Design review of the part built by this model. Coordinates are the model's own, in mm. Face numbers are marked on the shaded views. Round coordinates to 2 decimals unless told otherwise and drop trailing zeros. Order: outer loops, then holes, each group sorted by start corner. A loop starts at its lowest first (then second) coordinate and runs counter-clockwise, first axis right, second up. Notation, with made-up numbers: (26, 31) - (42, 31) arc R20 ccw to (42, 37) - close; hole circle Ø10 at (-32, 58). An arc over 180 degrees is marked (long way). Answer as a JSON object with one key per item and string values. Group by question number.
from build123d import *
from build123d import SkipClean  # not in build123d's __all__

# Parameters (mm, degrees)
F0_R      = 6.35
F1_DEPTH  = 25.4
F2_R      = 6.35
F3_DEPTH  = 25.4
F4_DEPTH  = 5.08
F5_DEPTH  = 8.89
F6_DEPTH  = 20.32
F7_DEPTH  = 10.16
F8_DEPTH  = 5.08
F9_DEPTH  = 13.97
F10_DEPTH = 3.81
F11_W     = 3.81
F11_H     = 6.35
F12_DEPTH = 6.35
F17_DEPTH = 2.032
F18_DEPTH = 2.032


with BuildPart() as f1:
    # F0 (on Front) → F1 (new body)
    with BuildSketch(Plane.XZ):
        with BuildLine():
            ThreePointArc((42.0866659097, -2.2684633732), (38.3669220307, 6.7117927479), (29.3866659097, 10.4315366268))
            ThreePointArc((29.3866659097, 10.4315366268), (20.4064097886, 6.7117927479), (16.6866659097, -2.2684633732))
            ThreePointArc((16.6866659097, -2.2684633732), (20.4064097886, -11.2487194943), (29.3866659097, -14.9684633732))
            ThreePointArc((29.3866659097, -14.9684633732), (38.3669220307, -11.2487194943), (42.0866659097, -2.2684633732))
        make_face()
        with Locations((29.3866659097, -2.2684633732)):
            Circle(F0_R, mode=Mode.SUBTRACT)
        with Locations((29.3866659097, -2.2684633732)):
            Circle(F0_R)
        with BuildLine():
            Line((92.8866659097, 10.4315366268), (29.3866659097, 10.4315366268))
            ThreePointArc((29.3866659097, 10.4315366268), (38.3669220307, 6.7117927479), (42.0866659097, -2.2684633732))
            ThreePointArc((42.0866659097, -2.2684633732), (38.3669220307, -11.2487194943), (29.3866659097, -14.9684633732))
            Line((29.3866659097, -14.9684633732), (92.8866659097, -14.9684633732))
            Line((92.8866659097, -14.9684633732), (92.8866659097, 10.4315366268))
        make_face()
    extrude(amount=-F1_DEPTH)

    # F2 (on face) → F3 (cut, through all)
    with BuildSketch(Plane(origin=(0, 25.4, 0), x_dir=(-1, 0, 0), z_dir=(0, 1, 0))):
        with BuildLine():
            ThreePointArc((-29.3866659097, -14.9684633732), (-42.0866659097, -2.2684633732), (-29.3866659097, 10.4315366268))
            Line((-29.3866659097, 10.4315366268), (-92.8866659097, 10.4315366268))
            Line((-92.8866659097, 10.4315366268), (-92.8866659097, -14.9684633732))
            Line((-92.8866659097, -14.9684633732), (-29.3866659097, -14.9684633732))
        make_face()
        with Locations((-29.3866659097, -2.2684633732)):
            Circle(F2_R)
    with SkipClean():  # cleaning this boolean's faces spoils the solid; the shape is the same uncleaned
        extrude(amount=-F3_DEPTH, mode=Mode.SUBTRACT)

    # F2 (on face) → F4 (join)
    with BuildSketch(Plane(origin=(0, 25.4, 0), x_dir=(-1, 0, 0), z_dir=(0, 1, 0))):
        with BuildLine():
            ThreePointArc((-29.3866659097, -14.9684633732), (-42.0866659097, -2.2684633732), (-29.3866659097, 10.4315366268))
            Line((-29.3866659097, 10.4315366268), (-92.8866659097, 10.4315366268))
            Line((-92.8866659097, 10.4315366268), (-92.8866659097, -14.9684633732))
            Line((-92.8866659097, -14.9684633732), (-29.3866659097, -14.9684633732))
        make_face()
    extrude(amount=-F4_DEPTH)

    # F2 (on face) → F5 (join)
    with BuildSketch(Plane(origin=(0, 25.4, 0), x_dir=(-1, 0, 0), z_dir=(0, 1, 0))):
        with Locations((-29.3866659097, -2.2684633732)):
            Circle(F2_R)
    extrude(amount=-F5_DEPTH)

    # F2 (on face) → F6 (join)
    with BuildSketch(Plane(origin=(0, 25.4, 0), x_dir=(-1, 0, 0), z_dir=(0, 1, 0))):
        with BuildLine():
            ThreePointArc((-29.3866659097, -14.9684633732), (-42.0866659097, -2.2684633732), (-29.3866659097, 10.4315366268))
            Line((-29.3866659097, 10.4315366268), (-92.8866659097, 10.4315366268))
            Line((-92.8866659097, 10.4315366268), (-92.8866659097, -14.9684633732))
            Line((-92.8866659097, -14.9684633732), (-29.3866659097, -14.9684633732))
        make_face()
        with Locations((-29.3866659097, -2.2684633732)):
            Circle(F2_R)
    extrude(amount=-F6_DEPTH)

    # F7 (cut): a face of the model
    f7_faces = [f1.faces().sort_by_distance(p)[0] for p in [
        (29.3866659097, 0, 10.072326382),
    ]]
    extrude(f7_faces, amount=-F7_DEPTH, mode=Mode.SUBTRACT)

    # F8 (cut): a face of the model
    f8_faces = [f1.faces().sort_by_distance(p)[0] for p in [
        (66.0488875518, 5.08, -2.2684633732),
    ]]
    extrude(f8_faces, amount=-F8_DEPTH, mode=Mode.SUBTRACT)

    # F0 (on Front) → F9 (cut)
    with BuildSketch(Plane.XZ):
        with Locations((29.3866659097, -2.2684633732)):
            Circle(F0_R)
    extrude(amount=-F9_DEPTH, mode=Mode.SUBTRACT)

    # F2 (on face) → F10 (cut)
    with BuildSketch(Plane(origin=(0, 25.4, 0), x_dir=(-1, 0, 0), z_dir=(0, 1, 0))):
        with Locations((-29.3866659097, -2.2684633732)):
            Circle(F2_R)
    extrude(amount=-F10_DEPTH, mode=Mode.SUBTRACT)

    # F11 (on face) → F12 (join)
    with BuildSketch(Plane.YZ.offset(92.8866659097)):
        with Locations((12.065, 7.2565366268)):
            Rectangle(F11_W, F11_H)
        with Locations((23.495, 7.2565366268)):
            Rectangle(F11_W, F11_H)
        with Locations((23.495, -11.7934633732)):
            Rectangle(F11_W, F11_H)
        with Locations((12.065, -11.7934633732)):
            Rectangle(F11_W, F11_H)
    extrude(amount=F12_DEPTH)

    # F15 (on face) + F13 (on face) → F17 (join)
    with BuildSketch(Plane(origin=(0, 13.97, 0), x_dir=(-1, 0, 0), z_dir=(0, 1, 0))):
        with BuildLine():
            Line((-96.0616659097, -11.7934633732), (-94.1566659097, -11.7934633732))
            ThreePointArc((-94.1566659097, -11.7934633732), (-94.7146274915, -10.446424955), (-96.0616659097, -9.8884633732))
            Line((-96.0616659097, -9.8884633732), (-96.0616659097, -11.7934633732))
        make_face()
        with BuildLine():
            Line((-97.9666659097, -11.7934633732), (-96.0616659097, -11.7934633732))
            Line((-96.0616659097, -11.7934633732), (-96.0616659097, -9.8884633732))
            ThreePointArc((-96.0616659097, -9.8884633732), (-97.4087043278, -10.446424955), (-97.9666659097, -11.7934633732))
        make_face()
        with BuildLine():
            Line((-96.0616659097, -13.6984633732), (-96.0616659097, -11.7934633732))
            Line((-96.0616659097, -11.7934633732), (-97.9666659097, -11.7934633732))
            ThreePointArc((-97.9666659097, -11.7934633732), (-97.4087043278, -13.1405017913), (-96.0616659097, -13.6984633732))
        make_face()
        with BuildLine():
            ThreePointArc((-96.0616659097, -13.6984633732), (-94.7146274915, -13.1405017913), (-94.1566659097, -11.7934633732))
            Line((-94.1566659097, -11.7934633732), (-96.0616659097, -11.7934633732))
            Line((-96.0616659097, -11.7934633732), (-96.0616659097, -13.6984633732))
        make_face()
    with BuildSketch(Plane(origin=(0, 13.97, 0), x_dir=(-1, 0, 0), z_dir=(0, 1, 0))):
        with BuildLine():
            Line((-96.0616659097, 7.2565366268), (-96.0616659097, 9.1615366268))
            ThreePointArc((-96.0616659097, 9.1615366268), (-97.4087043278, 8.603575045), (-97.9666659097, 7.2565366268))
            Line((-97.9666659097, 7.2565366268), (-96.0616659097, 7.2565366268))
        make_face()
        with BuildLine():
            Line((-96.0616659097, 7.2565366268), (-94.1566659097, 7.2565366268))
            ThreePointArc((-94.1566659097, 7.2565366268), (-94.7146274915, 8.603575045), (-96.0616659097, 9.1615366268))
            Line((-96.0616659097, 9.1615366268), (-96.0616659097, 7.2565366268))
        make_face()
        with BuildLine():
            ThreePointArc((-97.9666659097, 7.2565366268), (-97.4087043278, 5.9094982087), (-96.0616659097, 5.3515366268))
            Line((-96.0616659097, 5.3515366268), (-96.0616659097, 7.2565366268))
            Line((-96.0616659097, 7.2565366268), (-97.9666659097, 7.2565366268))
        make_face()
        with BuildLine():
            ThreePointArc((-96.0616659097, 5.3515366268), (-94.7146274915, 5.9094982087), (-94.1566659097, 7.2565366268))
            Line((-94.1566659097, 7.2565366268), (-96.0616659097, 7.2565366268))
            Line((-96.0616659097, 7.2565366268), (-96.0616659097, 5.3515366268))
        make_face()
    extrude(amount=F17_DEPTH)

    # F14 (on face) + F16 (on face) → F18 (join)
    with BuildSketch(Plane.XZ.offset(-21.59)):
        with BuildLine():
            Line((96.0616659097, 7.2565366268), (96.0616659097, 9.1615366268))
            ThreePointArc((96.0616659097, 9.1615366268), (94.7146274915, 8.603575045), (94.1566659097, 7.2565366268))
            Line((94.1566659097, 7.2565366268), (96.0616659097, 7.2565366268))
        make_face()
        with BuildLine():
            Line((96.0616659097, 7.2565366268), (97.9666659097, 7.2565366268))
            ThreePointArc((97.9666659097, 7.2565366268), (97.4087043278, 8.603575045), (96.0616659097, 9.1615366268))
            Line((96.0616659097, 9.1615366268), (96.0616659097, 7.2565366268))
        make_face()
        with BuildLine():
            ThreePointArc((96.0616659097, 5.3515366268), (97.4087043278, 5.9094982087), (97.9666659097, 7.2565366268))
            Line((97.9666659097, 7.2565366268), (96.0616659097, 7.2565366268))
            Line((96.0616659097, 7.2565366268), (96.0616659097, 5.3515366268))
        make_face()
        with BuildLine():
            ThreePointArc((94.1566659097, 7.2565366268), (94.7146274915, 5.9094982087), (96.0616659097, 5.3515366268))
            Line((96.0616659097, 5.3515366268), (96.0616659097, 7.2565366268))
            Line((96.0616659097, 7.2565366268), (94.1566659097, 7.2565366268))
        make_face()
    with BuildSketch(Plane.XZ.offset(-21.59)):
        with BuildLine():
            Line((94.1566659097, -11.7934633732), (96.0616659097, -11.7934633732))
            Line((96.0616659097, -11.7934633732), (96.0616659097, -9.8884633732))
            ThreePointArc((96.0616659097, -9.8884633732), (94.7146274915, -10.446424955), (94.1566659097, -11.7934633732))
        make_face()
        with BuildLine():
            Line((96.0616659097, -9.8884633732), (96.0616659097, -11.7934633732))
            Line((96.0616659097, -11.7934633732), (97.9666659097, -11.7934633732))
            ThreePointArc((97.9666659097, -11.7934633732), (97.4087043278, -10.446424955), (96.0616659097, -9.8884633732))
        make_face()
        with BuildLine():
            Line((96.0616659097, -11.7934633732), (96.0616659097, -13.6984633732))
            ThreePointArc((96.0616659097, -13.6984633732), (97.4087043278, -13.1405017913), (97.9666659097, -11.7934633732))
            Line((97.9666659097, -11.7934633732), (96.0616659097, -11.7934633732))
        make_face()
        with BuildLine():
            ThreePointArc((94.1566659097, -11.7934633732), (94.7146274915, -13.1405017913), (96.0616659097, -13.6984633732))
            Line((96.0616659097, -13.6984633732), (96.0616659097, -11.7934633732))
            Line((96.0616659097, -11.7934633732), (94.1566659097, -11.7934633732))
        make_face()
    extrude(amount=F18_DEPTH)


solid = f1.part
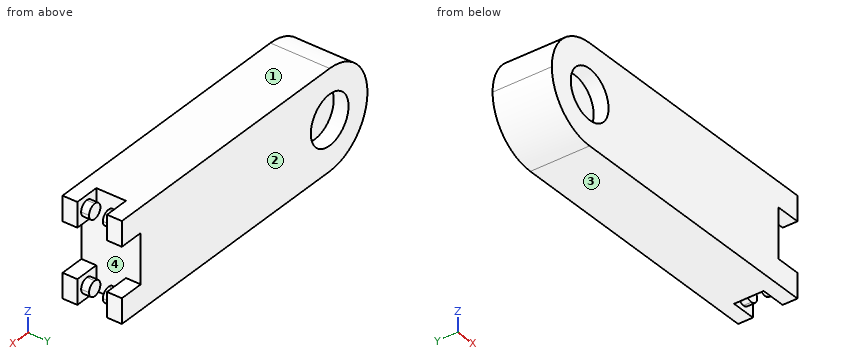
1. Clearance check with flat-ended pins moving along their axes: P1, Ø4.5, axis at y = 16, z = -5.5, coming from the +X side; P2, Ø4, axis at x = 27, y = 13.5, coming from the -Z side; P3, Ø10, axis at x = 29.39, z = -2.27, coming from the -Y side. State where each tip first meets the part, or that it passes through.
2. Take a section at D-D, the plane x = 33. Give the boundary of the cut face in (y, z).
3. Mouldability with a two-part tool opening along Z and no side actions: class the marked faces 1, 2, 3 and 4 as pulls with the +Z half, pulls with the -Z half, needs draft (parallel to the pull), parting line crosses it, or undercut.
4. Take a section at C-C, the plane z = -3. Give the boundary of the cut face in (x, y), then the cut area to 3 significant figures.
5. To check wall thickness, follow line 1 (X direction, y = 19, z = -1.75); line 2 (Y direction, x = 28.5, z = -6.25); line 3 (Z direction, x = 25, y = 24.5). State the ranges of each line that lie inside material, in increasing order. Write a range as from..to.
6. Take a section at B-B, the plane y = 17.5. Give the boundary of the cut face in (x, z).
7. Take a section at A-A, the plane y = 23. Give the boundary of the cut face in (x, z).
Response values:
{
 "1": {"P1": "x = 92.89", "P2": "z = -14.96", "P3": "y = 13.97"},
 "2": {"outline": "(10.16, -14.97) - (25.4, -14.97) - (25.4, -7.49) - (21.59, -7.49) - (21.59, 2.95) - (25.4, 2.95) - (25.4, 10.43) - (10.16, 10.43) - (10.16, 2.95) - (13.97, 2.95) - (13.97, -7.49) - (10.16, -7.49) - close"},
 "3": {"face 1": "pulls with the +Z half", "face 2": "needs draft", "face 3": "pulls with the -Z half", "face 4": "undercut"},
 "4": {"outline": "(16.71, 10.16) - (23.08, 10.16) - (23.08, 13.97) - (35.69, 13.97) - (35.69, 10.16) - (92.89, 10.16) - (92.89, 25.4) - (35.69, 25.4) - (35.69, 21.59) - (23.08, 21.59) - (23.08, 25.4) - (16.71, 25.4) - close", "area": "1,060 mm2"},
 "5": {"line 1": "16.7..92.89", "line 2": "13.97..21.59", "line 3": "-14.19..-6.86, 2.32..9.65"},
 "6": {"outline": "(29.39, -14.97) - (92.89, -14.97) - (92.89, 10.43) - (29.39, 10.43) arc R12.7 ccw to start"},
 "7": {"outline": "(29.39, -14.97) - (99.24, -14.97) - (99.24, -8.62) - (92.89, -8.62) - (92.89, 4.08) - (99.24, 4.08) - (99.24, 10.43) - (29.39, 10.43) arc R12.7 ccw to start; hole circle Ø12.7 at (29.39, -2.27)"}
}
